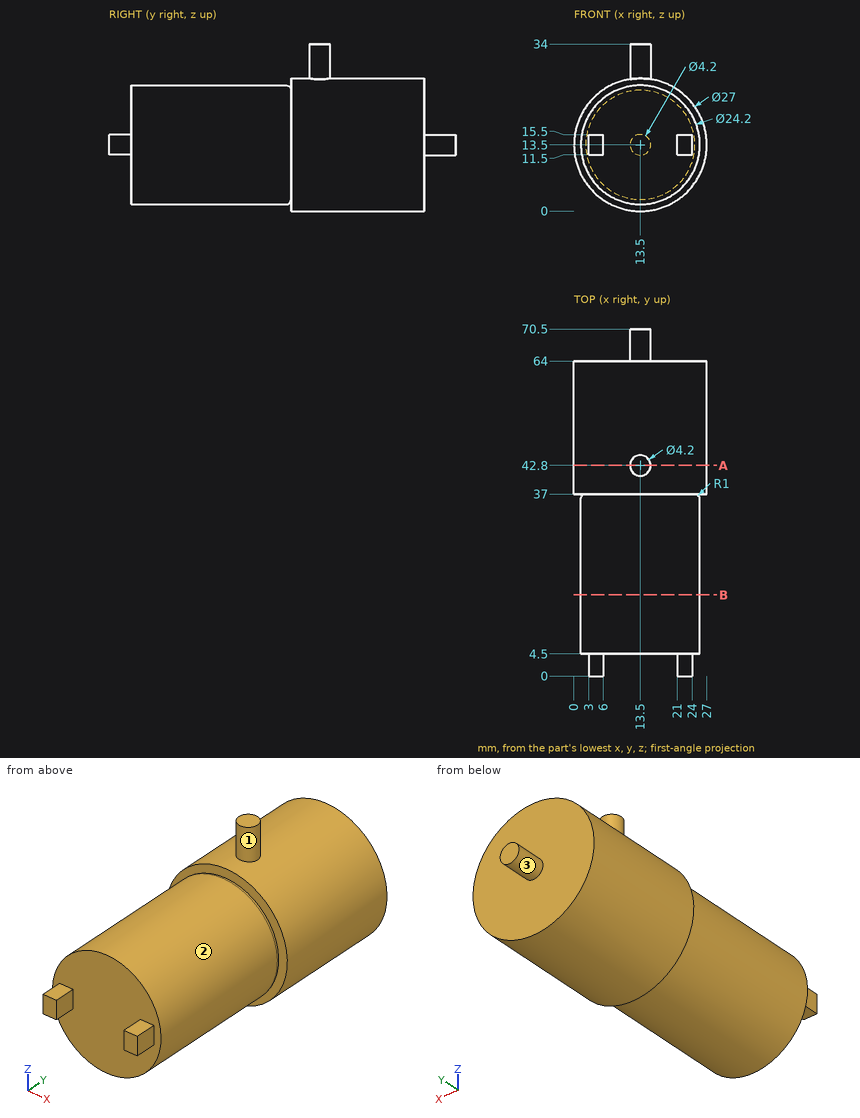
Study the drawing (mm; zero at the part's minimum x, y, z) and answer. A direction names the side the tool comes from. Give positions to 0.01 mm unless a question says otherwise; leave off trailing zeros. Write each loop counter-clockwise with the first axis right and the second up, starting at its lowest first coordinate (ties: lowest second). Pieces come first, ordered by that corner, then holes.
(1) The part is cut by section B-B on y = 16.5. Write down the section's boundary in (x, z).
Final values:
outline: circle Ø24.2 at (13.5, 13.5)
(2) Which of the six approach directions +Z, -Z, +X, -X, +Y, -Y give full straight-line access (tool end or side, diameter ignored) to the marked faces 1, 2 and 3?
Final values:
face 1: +Z
face 2: -Y
face 3: +Y
(3) Straight lines are drawn through the part: line 1 (Y direction, x = 22.25, z = 16); line 2 (Z direction, x = 14, y = 41.5); line 3 (X direction, y = 22, z = 13.5). For each, find the intervals that lie inside material, in ascending order.
Final values:
line 1: y = 4.5 to 64
line 2: z = 0.01 to 34
line 3: x = 1.4 to 25.6
(4) Flat-ended cylindrical pins translate along their axes: pin 1 Ø1 at (x, y) = (17.5, 12) entering from +Z; pin 2 Ø5 at (x, z) = (5.5, 4) entering from +Y; pin 3 Ø4.5 at (y, z) = (1.5, 13) entering from +X. Find the tip coordinate at first contact, or state that the pin passes through.
Final values:
pin 1: stops at z = 25.08
pin 2: stops at y = 64
pin 3: stops at x = 24
(5) The part is cut by section A-A on y = 42.8. Write down the section's boundary in (x, z).
Final values:
outline: (11.4, 26.84) arc R13.5 ccw (long way) to (15.6, 26.84) - (15.6, 34) - (11.4, 34) - close
